from build123d import *

# Parameters (mm, degrees)
F0_W     = 127
F0_H     = 101.6
F0_R     = 3.9878
F1_DEPTH = 9.525


with BuildPart() as f1:
    # F0 (on Top) → F1 (new body)
    with BuildSketch(Plane.XY):
        with Locations((63.5, 50.8)):
            Rectangle(F0_W, F0_H)
        with BuildLine():
            ThreePointArc((14.988244, 54.040302), (12.545255, 55.7418), (10.293505, 57.689338))
            ThreePointArc((10.293505, 57.689338), (10.180615, 63.345065), (15.836343, 63.457955))
            ThreePointArc((15.836343, 63.457955), (17.454745, 62.0582), (19.210594, 60.835283))
            ThreePointArc((19.210594, 60.835283), (20.496909, 55.326617), (14.988244, 54.040302))
        make_face(mode=Mode.SUBTRACT)
        with BuildLine():
            ThreePointArc((45.011756, 54.040302), (39.503091, 55.326617), (40.789406, 60.835283))
            ThreePointArc((40.789406, 60.835283), (42.545255, 62.0582), (44.163657, 63.457955))
            ThreePointArc((44.163657, 63.457955), (49.819385, 63.345065), (49.706495, 57.689338))
            ThreePointArc((49.706495, 57.689338), (47.454745, 55.7418), (45.011756, 54.040302))
        make_face(mode=Mode.SUBTRACT)
        with BuildLine():
            ThreePointArc((10.482321, 89.24346), (11.743749, 91.223108), (13.205196, 93.060056))
            ThreePointArc((13.205196, 93.060056), (18.85153, 93.404885), (19.19636, 87.758551))
            ThreePointArc((19.19636, 87.758551), (18.256251, 86.576892), (17.444809, 85.303439))
            ThreePointArc((17.444809, 85.303439), (11.993555, 83.792206), (10.482321, 89.24346))
        make_face(mode=Mode.SUBTRACT)
        with Locations((30, 78.198548)):
            Circle(F0_R, mode=Mode.SUBTRACT)
        with BuildLine():
            ThreePointArc((40.80364, 87.758551), (41.14847, 93.404885), (46.794804, 93.060056))
            ThreePointArc((46.794804, 93.060056), (48.256251, 91.223108), (49.517679, 89.24346))
            ThreePointArc((49.517679, 89.24346), (48.006445, 83.792206), (42.555191, 85.303439))
            ThreePointArc((42.555191, 85.303439), (41.743749, 86.576892), (40.80364, 87.758551))
        make_face(mode=Mode.SUBTRACT)
    extrude(amount=F1_DEPTH)


solid = f1.part
Verification items for the finished model (mm, model axes). A direction names the side the tool comes from. Coordinates: 2 decimals unless noted, no trailing zeros. Loops run counter-clockwise (first coordinate to the right, second up) from the corner with the lowest first, then second, coordinate; pieces in that order, holes last. Notation, with made-up numbers: (73.5, 76.5) -> (117.5, 76.5) arc R20 cw to (117.5, 87.5) -> close; hole circle Ø2 at (23, 18). An arc over 180 degrees is marked (long way). Write each question's results on one line, items separated by ' | '.
Item 1: Mould release check, pull along Y, two halves, no side actions. Record for faces 3 (the face through (48.083, 83.836, 4.696)), 4 (the face through (63, 0, 5)), 5 (the face through (63, 52, 9.525)), 6 (the face through (63, 101.6, 5)): +Y half, -Y half, draft (parallel to the pull), parting line (faces both ways), or undercut.
Found:
face 3: undercut | face 4: -Y half | face 5: draft | face 6: +Y half
Item 2: Section check B-B, the plane z = 4.5. Enter the section's corners in (x, y), plus the area to 3 significant figures.
Found:
outline: (0, 0) -> (127, 0) -> (127, 101.6) -> (0, 101.6) -> close; hole (10.29, 57.69) arc R28.44 ccw to (14.99, 54.04) arc R4 ccw to (19.21, 60.84) arc R20.44 cw to (15.84, 63.46) arc R4 ccw to start; hole (10.48, 89.24) arc R4 ccw to (17.44, 85.3) arc R14.43 cw to (19.2, 87.76) arc R4 ccw to (13.21, 93.06) arc R22.43 ccw to start; hole circle Ø7.98 at (30, 78.2); hole (40.79, 60.84) arc R4 ccw to (45.01, 54.04) arc R28.44 ccw to (49.71, 57.69) arc R4 ccw to (44.16, 63.46) arc R20.44 cw to start; hole (40.8, 87.76) arc R14.43 cw to (42.56, 85.3) arc R4 ccw to (49.52, 89.24) arc R22.43 ccw to (46.79, 93.06) arc R4 ccw to start | area: 12,500 mm2
Item 3: Section check A-A, the plane x = 30. Enter the section's corners in (y, z) (3 decimals).
Found:
outline: (0, 0) -> (74.211, 0) -> (74.211, 9.525) -> (0, 9.525) -> close; (82.186, 0) -> (101.6, 0) -> (101.6, 9.525) -> (82.186, 9.525) -> close
Item 4: Material ranges on L1, parallel to X at y = 57.5, z = 6; L2, parallel to Y at x = 30, z = 3.5; L3, parallel to X at y = 58, z = 1.5, recorded low to high.
Found:
L1: x = 0 to 10.49, 21.1 to 38.9, 49.51 to 127 | L2: y = 0 to 74.21, 82.19 to 101.6 | L3: x = 0 to 10, 21.06 to 38.94, 50 to 127
Item 5: Tool access check on faces 1 (the face through (48.237, 91.25, 4.696)), 2 (the face through (0, 50, 5)). Record the directions out of +Z, -Z, +X, -X, +Y, -Y that give a thin tool (end or side, any length) a straight path to the whole face; none if there is none.
Found:
face 1: +Z, -Z | face 2: +Z, -Z, -X, +Y, -Y
